Could you check a few things on this model? Use its own coordinates, in mm. A direction names the side the tool comes from. Round coordinates to 2 decimals unless told otherwise and drop trailing zeros. Loops run counter-clockwise (first coordinate to the right, second up) from the corner with the lowest first, then second, coordinate; pieces in that order, holes last. Notation, with made-up numbers: (43.5, 22) -> (84.5, 22) arc R15 cw to (84.5, 44) -> close; hole circle Ø5 at (0.5, 3.25). An arc over 180 degrees is marked (long way). One line per item, written item: value.
```python
from build123d import *

# Parameters (mm, degrees)
F1_DEPTH = 2000
F2_R     = 6
F3_DEPTH = 488.001


with BuildPart() as f1:
    # F0 (on Top) → F1 (new body)
    with BuildSketch(Plane.XY):
        with BuildLine():
            ThreePointArc((238, 0), (0, -238), (-238, 0))
            Line((-238, 0), (-238, 60))
            Line((-238, 60), (-244, 60))
            Line((-244, 60), (-244, 0))
            ThreePointArc((-244, 0), (0, -244), (244, 0))
            Line((244, 0), (244, 60))
            Line((244, 60), (238, 60))
            Line((238, 60), (238, 0))
        make_face()
    extrude(amount=F1_DEPTH)

    # F2 (on face) → F3 (cut, through all)
    with BuildSketch(Plane.YZ.offset(244)):
        with Locations((30, 1750)):
            Circle(F2_R)
        with Locations((30, 1250)):
            Circle(F2_R)
        with Locations((30, 750)):
            Circle(F2_R)
        with Locations((30, 250)):
            Circle(F2_R)
    extrude(amount=-F3_DEPTH, mode=Mode.SUBTRACT)


solid = f1.part
```
(1) We'd pull the mould along X, two halves only. Please class faces 1 (the face through (5.233, -237.942, 986)), 2 (the face through (-5.37, -243.94, 986)), 3 (the face through (-244, 30, 986)), 4 (the face through (-238, 30, 986)): +X half, -X half, draft (parallel to the pull), parting line (faces both ways), or undercut.
Results below:
face 1: undercut
face 2: parting line
face 3: -X half
face 4: undercut
(2) Imagine slicing it at B-B on z = 1806. Write out the boundary of the cut face in (x, y).
Results below:
outline: (-244, 0) arc R244 ccw to (244, 0) -> (244, 60) -> (238, 60) -> (238, 0) arc R238 cw to (-238, 0) -> (-238, 60) -> (-244, 60) -> close
(3) On a 3-axis mill with a long thin cutter (end or side, diameter ignored), from which of +Z, -Z, +X, -X, +Y, -Y can I reach the whole of each face in a straight line? I mean faces 5 (the face through (17, -238, 0)), 6 (the face through (238, 30, 986)). Say none if no direction works.
Results below:
face 5: -Z, +X, -X, +Y, -Y
face 6: +Z, -Z, +Y
(4) For pin 1 Ø4 at (x, z) = (-169.5, 1326.5) entering from -Y; pin 2 Ø1 at (x, z) = (135.5, 1503) entering from -Y; pin 3 Ø8 at (x, z) = (125, 1683.5) entering from -Y; pin 4 Ø11 at (y, z) = (30, 1250) entering from +X, each with a flat end and sliding along its axis, tell me the tip position at first contact or that it passes through.
Results below:
pin 1: stops at y = -177.43
pin 2: stops at y = -203.25
pin 3: stops at y = -211.88
pin 4: passes through
(5) Please list where these lines run through material, in increasing order: L1, parallel to Z at x = 239.5, y = 30; L2, parallel to X at y = 35.5, z = 1239; L3, parallel to Y at x = 10, z = 1415 (3 decimals).
Results below:
L1: z = 0 to 244, 256 to 744, 756 to 1244, 1256 to 1744, 1756 to 2000
L2: x = -244 to -238, 238 to 244
L3: y = -243.795 to -237.79
(6) Imagine slicing it at A-A on y = -45. Write out the boundary of the cut face in (x, z), then the cut area to 3 significant figures.
Results below:
outline: (-239.81, 0) -> (-233.71, 0) -> (-233.71, 2000) -> (-239.81, 2000) -> close; (233.71, 0) -> (239.81, 0) -> (239.81, 2000) -> (233.71, 2000) -> close
area: 24,400 mm²
(7) Imagine slicing it at C-C on x = 0. Write out the boundary of the cut face in (y, z).
Results below:
outline: (-244, 0) -> (-238, 0) -> (-238, 2000) -> (-244, 2000) -> close
(8) Imagine slicing it at D-D on x = -181. Write out the boundary of the cut face in (y, z), then the cut area to 3 significant figures.
Results below:
outline: (-163.63, 0) -> (-154.54, 0) -> (-154.54, 2000) -> (-163.63, 2000) -> close
area: 18,200 mm²
